Autodesk Inventor part; units mm, degrees
ref_plane "YZ Plane" through (0, 0, 0) normal (1, 0, 0) x (0, 1, 0)
ref_plane "XZ Plane" through (0, 0, 0) normal (0, 1, 0) x (-1, 0, 0)
ref_plane "XY Plane" through (0, 0, 0) normal (0, 0, 1) x (1, 0, 0)
sketch "Sketch1" plane through (0, 0, 0) normal (0, 0, 1) x (1, 0, 0)
  line L0 (344.9937, 353.3773) -> (-355.0063, 353.3773)
  line L1 (-455.0063, 253.3773) -> (-455.0063, -46.6227)
  line L2 (-355.0063, -146.6227) -> (344.9937, -146.6227)
  line L3 (344.9937, -146.6227) -> (344.9937, 53.3773)
  line L4 (344.9937, 153.3773) -> (344.9937, 353.3773)
  arc A0 (-63.585, 153.3773) -> (-63.585, 53.3773) centre (-205.0063, 103.3773) ccw
  line L5 (344.9937, 153.3773) -> (-63.585, 153.3773)
  line L6 (344.9937, 53.3773) -> (-63.585, 53.3773)
  arc A1 (-355.0063, 353.3773) -> (-455.0063, 253.3773) centre (-355.0063, 253.3773) ccw
  arc A2 (-455.0063, -46.6227) -> (-355.0063, -146.6227) centre (-355.0063, -46.6227) ccw
  point P0 (0, 0)
  point P1 (-455.0063, 353.3773)
  point P2 (-455.0063, -146.6227)
  dimension "d0" = 800
  dimension "d1" = 500
  dimension "d8" = 250
  dimension "d9" = 300
  dimension "d10" = 100
  dimension "d11" = 100
  dimension "d12" = 200
  dimension "d13" = 200
extrude "Extrusion1" add sketch "Sketch1" along normal blind 500
sketch "Sketch2" plane through (-355.0063, 353.3773, 0) normal (0, 1, 0) x (1, 0, 0)
  circle A0 centre (500, -250) radius 112.7771
  line L0 (700, -500) -> (0, -500)
  line L1 (700, 0) -> (700, -500)
  point P0 (355.0063, 0)
  dimension "d16" = 250
  dimension "d17" = 200
extrude "Extrusion2" cut sketch "Sketch2" against normal blind 700
properties part number "BT15_Klemme"
Read the model definition and answer for the solid it produces. Units are mm, in the model's axes. A direction names the side the tool comes from. Round coordinates to 2 decimals unless told otherwise and drop trailing zeros. Write each loop counter-clockwise with the first axis right and the second up, starting at its lowest first coordinate (ties: lowest second). Pieces come first, ordered by that corner, then holes. Notation, with made-up numbers: M 5.25,40 L 17.25,40 A14 ccw 17.25,66 Z; hole C 26,-7.75 d9. An arc over 180 degrees is marked long. One line per item, written item: value.
Q1. Find section D-D on x = 137.5. Write down the section's boundary in (y, z), plus the area to 3 significant figures.
Data:
outline: M -146.62,0 L 53.38,0 L 53.38,137.47 L -146.62,137.47 Z; M -146.62,362.53 L 53.38,362.53 L 53.38,500 L -146.62,500 Z; M 153.38,0 L 353.38,0 L 353.38,137.47 L 153.38,137.47 Z; M 153.38,362.53 L 353.38,362.53 L 353.38,500 L 153.38,500 Z
area: 110,000 mm2
Q2. Find section C-C on z = 250. Write down the section's boundary in (x, y) (3 decimals), plus the area to 3 significant figures.
Data:
outline: M -455.006,-46.623 A100 ccw -355.006,-146.623 L 32.217,-146.623 L 32.217,53.377 L -63.585,53.377 A150 cw long -63.585,153.377 L 32.217,153.377 L 32.217,353.377 L -355.006,353.377 A100 ccw -455.006,253.377 Z; M 257.771,-146.623 L 344.994,-146.623 L 344.994,53.377 L 257.771,53.377 Z; M 257.771,153.377 L 344.994,153.377 L 344.994,353.377 L 257.771,353.377 Z
area: 195,000 mm2
Q3. Straight lines are drawn through the part: line 1 (Y direction, x = -212, z = 96.5); line 2 (X direction, y = -22, z = 264.5); line 3 (Y direction, x = 309, z = 474.5). For each, find the intervals that lie inside material, in ascending order. Write a range as [from, to].
Data:
line 1: [-146.62, -46.46], [253.21, 353.38]
line 2: [-455.01, -287.35], [-122.66, 33.15], [256.83, 344.99]
line 3: [-146.62, 53.38], [153.38, 353.38]
Q4. Which of the six approach directions +Z, -Z, +X, -X, +Y, -Y give full straight-line access (tool end or side, diameter ignored) to faces 4 (the flat face through (144, 53.377, 135)), 5 (the cylindrical face through (-426.49, 323.306, 246.5))?
Data:
face 4: +Z, -Z, +X
face 5: +Z, -Z, -X, +Y
Q5. Find section B-B on y = 29. Write down the section's boundary in (x, z).
Data:
outline: M -455.01,0 L -335.27,0 L -335.27,500 L -455.01,500 Z; M -74.75,0 L 344.99,0 L 344.99,500 L -74.75,500 Z; hole C 144.99,250 d225.55
Q6. Flat-ended cylindrical pins translate along their axes: pin 1 Ø4 at (y, z) = (77.5, 256.5) entering from +X; pin 2 Ø1 at (y, z) = (-56, 260) entering from -X. Find the tip coordinate at first contact, or state that the pin passes through.
Data:
pin 1: x = -352.39
pin 2: x = -454.61
Q7. Find section A-A on x = 288. Write down the section's boundary in (y, z).
Data:
outline: M -146.62,0 L 53.38,0 L 53.38,500 L -146.62,500 Z; M 153.38,0 L 353.38,0 L 353.38,500 L 153.38,500 Z
Q8. For a pull along X with two mould halves and no side action, classify faces 1 (the flat face through (0, 353.377, 246)), 2 (the cylindrical face through (55.498, -45.223, 318.623)), 3 (the flat face through (344.994, -48, 246)) as +X half, -X half, draft (parallel to the pull), parting line (faces both ways), or undercut.
Data:
face 1: draft
face 2: undercut
face 3: +X half
